Autodesk Inventor part; units mm, degrees
ref_plane "YZ Plane" through (0, 0, 0) normal (1, 0, 0) x (0, 1, 0)
ref_plane "XZ Plane" through (0, 0, 0) normal (0, 1, 0) x (-1, 0, 0)
ref_plane "XY Plane" through (0, 0, 0) normal (0, 0, 1) x (1, 0, 0)
sketch "スケッチ1" plane through (0, 0, 0) normal (1, 0, 0) x (0, 1, 0)
  line L0 (-6.5, 0) -> (6.5, 0)
  line L1 (0, 0) -> (0, 3.1754) construction
  line L2 (-6.2544, 3.1754) -> (-6.5, 2.75)
  line L3 (-6.5, 2.75) -> (-6.5, 0)
  line L4 (-6.2544, 3.1754) -> (6.2544, 3.1754)
  line L5 (6.2544, 3.1754) -> (6.5, 2.75)
  line L6 (6.5, 2.75) -> (6.5, 0)
  dimension "d1" = 2.75
  dimension "d2" = 3.1754
  dimension "d3" = 30
  dimension "d4" = 13
revolve "回転1" add sketch "スケッチ1" angle 360 about axis through (0, -6.5, 0) along (0, 1, 0)
sketch "スケッチ2" plane through (0, 6.5, 0) normal (0, 1, 0) x (1, 0, 0)
  circle A0 centre (0, 0) radius 3.1754
  line L0 (0, -3.1754) -> (-2.75, -1.5877)
  line L1 (-2.75, -1.5877) -> (-2.75, 1.5877)
  line L2 (-2.75, 1.5877) -> (0, 3.1754)
  line L3 (0, 3.1754) -> (2.75, 1.5877)
  line L4 (2.75, 1.5877) -> (2.75, -1.5877)
  line L5 (2.75, -1.5877) -> (0, -3.1754)
  point P0 (0, 0)
  point P1 (0, 0)
  point P2 (2.75, -1.5877)
  point P3 (2.75, -1.5877)
  point P4 (2.75, 1.5877)
  point P5 (2.75, 1.5877)
  point P6 (0, 3.1754)
  point P7 (0, 3.1754)
  point P8 (-2.75, 1.5877)
  point P9 (-2.75, 1.5877)
  point P10 (-2.75, -1.5877)
  point P11 (-2.75, -1.5877)
extrude "押し出し1" cut sketch "スケッチ2" against normal through all contours A0 L4 | L3 A0 | A0 L5 | L2 A0 | A0 L0 | L1 A0
hole "穴1" at (0, 6.5, 0) direction (0, -1, 0) diameter 2.459 end through all countersink diameter 3 countersink angle 90
mirror "ミラー1" about plane through (0, 0, 0) normal (0, 1, 0) of "穴1"
equation "\"d2\" = 1.1547 * d1"
properties part number "ASL-313BE" material "アルミニウム 2014-T4"
Input: part model. Units: mm. Frame: model coordinates. Coordinates: 2 decimals unless noted, no trailing zeros. Loops run counter-clockwise (first coordinate to the right, second up) from the corner with the lowest first, then second, coordinate; pieces in that order, holes last.
Q1. Section A-A, the plane y = -2. Return the cut outline in (x, z), and give its area (3 significant figures).
Results are:
outline: (-2.75, -1.59) - (0, -3.18) - (2.75, -1.59) - (2.75, 1.59) - (0, 3.18) - (-2.75, 1.59) - close; hole circle Ø2.46 at (0, 0)
area: 21.4 mm2
Q2. Contact query for a flat-ended pin moving along its axis: pin 1 (3 mm diameter, centred on x = 2, y = -2.5, fed in from +Z). Output: stop coordinate, or through.
Results are:
pin 1: stops at z = 2.89
Q3. Line query: line 1 along X through (y, z) = (-2.5, 0); line 2 along X through (y, z) = (-1.5, 1); line 3 along Z through (x, y) = (-0.05, -5.25). Output: solid intervals per line, ascending.
Results are:
line 1: x = -2.75 to -1.23, 1.23 to 2.75
line 2: x = -2.75 to -0.72, 0.72 to 2.75
line 3: z = -3.15 to -1.23, 1.23 to 3.15
Q4. Mould query, pull axis X, two halves, no side actions, for faces 1 (the cylindrical face through (0.748, -0.087, -0.976)), 2 (the flat face through (-1.36, 0.09, 2.39)), 3 (the conical face through (2.52, 6.41, 1.44)). Classes: +X half, -X half, draft (parallel to the pull), parting line (faces both ways), or undercut.
Results are:
face 1: undercut
face 2: -X half
face 3: +X half
